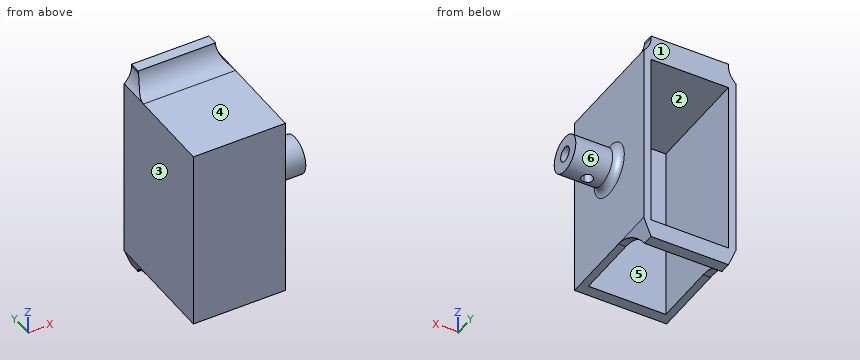
from build123d import *

# Parameters (mm, degrees)
BOSS_EXTRUDE1_DEPTH      = 29
BOSS_EXTRUDE1_DEPTH_BACK = 3
SKETCH1_W                = 25
SKETCH1_H                = 50
BOSS_EXTRUDE2_DEPTH      = 3
BOSS_EXTRUDE3_START      = 29
SKETCH1_4_W              = 21
SKETCH1_4_H              = 5
BOSS_EXTRUDE3_DEPTH      = 3
CUT_EXTRUDE1_DEPTH       = 29
FILLET1_START            = -12.900995056
FILLET1_DEPTH            = 2
FILLET1_START_2          = 10.099004944
FILLET1_2_DEPTH          = 2
FILLET1_START_3          = 16
FILLET1_3_DEPTH          = 10
FILLET2_R                = 6
SKETCH2_R                = 5
SKETCH2_R_2              = 2
BOSS_EXTRUDE4_DEPTH      = 12
CUT_EXTRUDE3_DEPTH       = 30
FILLET5_R                = 2


with BuildPart() as part:
    # Sketch1 → Boss-Extrude1 (new, two sides: drawn at the far end of the back side and taken through both)
    with BuildSketch(Plane(origin=(0, 0, 0), x_dir=(1, 0, 0), z_dir=(0, 1, 0)).offset(-BOSS_EXTRUDE1_DEPTH_BACK)):
        with Locations((-0.400995056, -2.5)):
            Rectangle(SKETCH1_W, SKETCH1_H)
    extrude(amount=BOSS_EXTRUDE1_DEPTH + BOSS_EXTRUDE1_DEPTH_BACK)

    # Sketch1<3> → Boss-Extrude2 (add)
    with BuildSketch(Plane(origin=(0, 0, 0), x_dir=(1, 0, 0), z_dir=(0, 1, 0))):
        Polygon((-10.900995056, 22.5), (-10.900995056, 20.5), (-10.900995056, -25.5), (10.099004944, -25.5), (10.099004944, 20.5), (10.099004944, 22.5), align=None)
    extrude(amount=-BOSS_EXTRUDE2_DEPTH)

    # Sketch1<4> → Boss-Extrude3 (add)
    with BuildSketch(Plane(origin=(0, 0, 0), x_dir=(1, 0, 0), z_dir=(0, 1, 0)).offset(BOSS_EXTRUDE3_START)):
        Polygon((-12.900995056, 22.5), (12.099004944, 22.5), (10.099004944, 27.5), (-10.900995056, 27.5), align=None)
        with Locations((-0.400995056, -30)):
            Rectangle(SKETCH1_4_W, SKETCH1_4_H)
    extrude(amount=-BOSS_EXTRUDE3_DEPTH)

    # Sketch1<5> → Cut-Extrude1 (cut)
    with BuildSketch(Plane(origin=(0, 0, 0), x_dir=(1, 0, 0), z_dir=(0, 1, 0))):
        Polygon((-10.900995056, 22.5), (10.099004944, 22.5), (10.099004944, 20.5), (10.099004944, -25.5), (-10.900995056, -25.5), (-10.900995056, 20.5), align=None)
    extrude(amount=CUT_EXTRUDE1_DEPTH, mode=Mode.SUBTRACT)

    # Fillet1: read off the stored shape, not the designer's step
    # Fillet1 outline → Fillet1 (add)
    with BuildSketch(Plane.YZ.offset(FILLET1_START)):
        with BuildLine():
            ThreePointArc((17.339745962, -22.5), (22.339745962, -23.839745962), (26, -27.5))
            Line((26, -27.5), (26, -22.5))
            Line((26, -22.5), (17.339745962, -22.5))
        make_face()
    extrude(amount=FILLET1_DEPTH)

    # Fillet1 2 outline → Fillet1 2 (add)
    with BuildSketch(Plane.YZ.offset(FILLET1_START_2)):
        with BuildLine():
            ThreePointArc((17.339745962, -22.5), (22.339745962, -23.839745962), (26, -27.5))
            Line((26, -27.5), (26, -22.5))
            Line((26, -22.5), (17.339745962, -22.5))
        make_face()
    extrude(amount=FILLET1_2_DEPTH)

    # Fillet1 3 outline → Fillet1 3 (cut)
    with BuildSketch(Plane(origin=(0, 0, 0), x_dir=(1, 0, 0), z_dir=(0, 1, 0)).offset(FILLET1_START_3)):
        Polygon((-13.500995056, 21), (-10.300995056, 29), (-14, 29), (-14, 21), align=None)
        Polygon((14, 29), (9.499004944, 29), (12.699004944, 21), (14, 21), align=None)
    extrude(amount=FILLET1_3_DEPTH, mode=Mode.SUBTRACT)

    # Fillet2
    # the kernel refuses this fillet: 6 mm, written as the material it adds along each edge
    with BuildSketch(Plane(origin=(10.099004944, 26, 27.5), x_dir=(0, 0, 1), z_dir=(-1, 0, 0))) as fillet2_piece_1:
        with BuildLine():
            CenterArc((6, -5.916079783), FILLET2_R, 99.594068227, 80.405931773)
            Line((0, -5.916079783), (0, 0))
            Line((0, 0), (5, 0))
        make_face()
    extrude(amount=21)
    with BuildSketch(Plane(origin=(10.099004944, 29, 27.5), x_dir=(0, 0, 1), z_dir=(0, -1, 0))) as fillet2_piece_2:
        with BuildLine():
            CenterArc((4.472135955, -6), FILLET2_R, 90, 48.189685104)
            Line((0, -2), (0, 0))
            Line((0, 0), (4.472135955, 0))
        make_face()
    extrude(amount=3)
    with BuildSketch(Plane(origin=(-10.900995056, 29, 27.5), x_dir=(0, 0, 1), z_dir=(0, -1, 0))) as fillet2_piece_3:
        with BuildLine():
            CenterArc((4.472135955, 6), FILLET2_R, 221.810314896, 48.189685104)
            Line((0, 2), (0, 0))
            Line((0, 0), (4.472135955, 0))
        make_face()
    extrude(amount=3)
    with BuildSketch(Plane(origin=(24.889204401, 26, 27.5), x_dir=(0, 0, 1), z_dir=(-1, 0, 0))) as fillet2_piece_4a_section:
        with BuildLine():
            CenterArc((6, -5.916079783), FILLET2_R, 99.594068227, 80.405931773)
            Line((0, -5.916079783), (0, 0))
            Line((0, 0), (5, 0))
        make_face()
    fillet2_piece_4a = extrude(amount=35.790199458, mode=Mode.PRIVATE)
    fillet2_piece_4a = split(fillet2_piece_4a, bisect_by=Plane(origin=(12.099004944, 26, 27.5), z_dir=(-1, 0, 0)), keep=Keep.TOP, mode=Mode.PRIVATE)
    fillet2_piece_4a = split(fillet2_piece_4a, bisect_by=Plane(origin=(10.099004944, 26, 27.5), z_dir=(1, 0, 0)), keep=Keep.TOP, mode=Mode.PRIVATE)
    with BuildSketch(Plane(origin=(10.099004944, 29, 27.5), x_dir=(0, 0, 1), z_dir=(0, -1, 0))) as fillet2_piece_4b_section:
        with BuildLine():
            CenterArc((4.472135955, -6), FILLET2_R, 90, 48.189685104)
            Line((0, -2), (0, 0))
            Line((0, 0), (4.472135955, 0))
        make_face()
    fillet2_piece_4b = extrude(amount=14.180339887, mode=Mode.PRIVATE)
    fillet2_piece_4b = split(fillet2_piece_4b, bisect_by=Plane(origin=(10.099004944, 26, 27.5), z_dir=(0, -1, 0)), keep=Keep.TOP, mode=Mode.PRIVATE)
    fillet2_piece_4 = fillet2_piece_4a & fillet2_piece_4b
    add(fillet2_piece_4)
    with BuildSketch(Plane(origin=(-10.900995056, 29, 27.5), x_dir=(0, 0, 1), z_dir=(0, -1, 0))) as fillet2_piece_5a_section:
        with BuildLine():
            CenterArc((4.472135955, 6), FILLET2_R, 221.810314896, 48.189685104)
            Line((0, 2), (0, 0))
            Line((0, 0), (4.472135955, 0))
        make_face()
    fillet2_piece_5a = extrude(amount=14.180339887, mode=Mode.PRIVATE)
    fillet2_piece_5a = split(fillet2_piece_5a, bisect_by=Plane(origin=(-10.900995056, 26, 27.5), z_dir=(0, -1, 0)), keep=Keep.TOP, mode=Mode.PRIVATE)
    with BuildSketch(Plane(origin=(10.099004944, 26, 27.5), x_dir=(0, 0, 1), z_dir=(-1, 0, 0))) as fillet2_piece_5b_section:
        with BuildLine():
            CenterArc((6, -5.916079783), FILLET2_R, 99.594068227, 80.405931773)
            Line((0, -5.916079783), (0, 0))
            Line((0, 0), (5, 0))
        make_face()
    fillet2_piece_5b = extrude(amount=35.790199458, mode=Mode.PRIVATE)
    fillet2_piece_5b = split(fillet2_piece_5b, bisect_by=Plane(origin=(-12.900995056, 26, 27.5), z_dir=(1, 0, 0)), keep=Keep.TOP, mode=Mode.PRIVATE)
    fillet2_piece_5b = split(fillet2_piece_5b, bisect_by=Plane(origin=(-10.900995056, 26, 27.5), z_dir=(-1, 0, 0)), keep=Keep.TOP, mode=Mode.PRIVATE)
    fillet2_piece_5 = fillet2_piece_5a & fillet2_piece_5b
    add(fillet2_piece_5)

    # Sketch2 → Boss-Extrude4 (add)
    with BuildSketch(Plane(origin=(12.099004944, 0, 0), x_dir=(0, 0, -1), z_dir=(1, 0, 0))):
        with Locations(Location((-2.5, 13, 0), (0, 0, 180))):
            Circle(SKETCH2_R)
        with Locations((-2.5, 13)):
            Circle(SKETCH2_R_2, mode=Mode.SUBTRACT)
    extrude(amount=BOSS_EXTRUDE4_DEPTH)

    # Sketch3 → Cut-Extrude3 (cut)
    with BuildSketch(Plane.XY.offset(27.5)):
        with BuildLine():
            ThreePointArc((19.599004944, 13), (19.159665115, 14.060660172), (18.099004944, 14.5))
            Line((18.099004944, 14.5), (18.099004944, 11.5))
            ThreePointArc((18.099004944, 11.5), (19.159665115, 11.939339828), (19.599004944, 13))
        make_face()
        with BuildLine():
            Line((18.099004944, 11.5), (18.099004944, 14.5))
            ThreePointArc((18.099004944, 14.5), (16.599004944, 13), (18.099004944, 11.5))
        make_face()
    extrude(amount=-CUT_EXTRUDE3_DEPTH, mode=Mode.SUBTRACT)

    # Fillet5
    fillet5_edges = [part.edges().sort_by_distance(p)[0] for p in [
        (12.099004944, 13, -2.5),
    ]]
    fillet(fillet5_edges, radius=FILLET5_R)


solid = part.part
Here's how the part is built. I have some questions about the finished solid (model axes, mm). Face numbers are marked on the shaded views. A direction names the side the tool comes from. Round coordinates to 2 decimals unless told otherwise and drop trailing zeros. Order: outer loops, then holes, each group sorted by start corner. A loop starts at its lowest first (then second) coordinate and runs counter-clockwise, first axis right, second up. Notation, with made-up numbers: (-30, -25.5) -> (-5, -25.5) arc R16 cw to (-5, -11.5) -> close; hole circle Ø8 at (18, 30.25). An arc over 180 degrees is marked (long way). Return JSON: item names as keys, results as strings.
Q1. If we section it at C-C on y = 5: List the corners of the cut face in (x, z) for me.
Filled sheet:
{"outline": "(-12.9, -22.5) -> (-10.9, -22.5) -> (-10.9, 25.5) -> (10.1, 25.5) -> (10.1, -22.5) -> (12.1, -22.5) -> (12.1, 27.5) -> (-12.9, 27.5) -> close"}
Q2. If we section it at D-D on z = 11: List the corners of the cut face in (x, y) for me.
Filled sheet:
{"outline": "(-12.9, -3) -> (12.1, -3) -> (12.1, 29) -> (10.1, 29) -> (10.1, 0) -> (-10.9, 0) -> (-10.9, 29) -> (-12.9, 29) -> close"}
Q3. I need wall thicknesses on line 1 along X through (y, z) = (3.5, -21); line 2 along Y through (x, z) = (15.5, 2.5); line 3 along Z through (x, y) = (16.25, 13). Which ranges of each line are inside material? Lowest first, please. Write a range as from..to.
Filled sheet:
{"line 1": "x = -12.9..-10.9, 10.1..12.1", "line 2": "y = 8..11, 15..18", "line 3": "z = -2.5..0.5, 4.5..7.5"}
Q4. If we section it at A-A on x = 9: List the corners of the cut face in (y, z) for me, plus the area to 3 significant figures.
Filled sheet:
{"outline": "(-3, -22.5) -> (0, -22.5) -> (0, 25.5) -> (29, 25.5) -> (29, 32.5) -> (26, 32.5) arc R6 cw to (20.08, 27.5) -> (-3, 27.5) -> close; (26, -27.5) -> (29, -27.5) -> (29, -22.5) -> (26, -22.5) -> close", "area": "245 mm^2"}
Q5. If we mould it in two halves opening along X, with no side actions, what happens to the marked faces 1, 2 and 3? For each: released by +X, released by -X, zero draft, split by the parting line, or undercut.
Filled sheet:
{"face 1": "zero draft", "face 2": "undercut", "face 3": "released by -X"}
Q6. Which directions (+Z, -Z, +X, -X, +Y, -Y) give clear straight access to the entire face, cutting with the end or side of a thin tool? Please do the marked faces 4, 5 and 6.
Filled sheet:
{"face 4": "+Z, +X, -X, -Y", "face 5": "-Z, +Y", "face 6": "+X"}
Q7. If we section it at B-B on z = 2.5: List the corners of the cut face in (x, y) for me, plus the area to 3 significant figures.
Filled sheet:
{"outline": "(-12.9, -3) -> (12.1, -3) -> (12.1, 6) arc R2 cw to (14.1, 8) -> (24.1, 8) -> (24.1, 11) -> (12.1, 11) -> (12.1, 15) -> (24.1, 15) -> (24.1, 18) -> (14.1, 18) arc R2 cw to (12.1, 20) -> (12.1, 29) -> (10.1, 29) -> (10.1, 0) -> (-10.9, 0) -> (-10.9, 29) -> (-12.9, 29) -> close", "area": "265 mm^2"}
Q8. For pin 1 Ø1 at (x, z) = (12.5, -18.5) entering from +Y; pin 2 Ø10.5 at (x, y) = (2.5, 19.5) entering from -Z; pin 3 Ø10 at (x, y) = (20, 11) entering from -Z; pin 4 Ø16.5 at (x, y) = (1, 6) entering from -Z, each with a flat end and sliding along its axis, tell me the tip position at first contact or that it passes through.
Filled sheet:
{"pin 1": "stops at y = 29", "pin 2": "stops at z = 25.5", "pin 3": "stops at z = -2.5", "pin 4": "stops at z = -22.5"}
